Can you work these out from the model? Positions are in its coordinate system, mm. A direction names the side the tool comes from. Round coordinates to 2 decimals unless told otherwise and drop trailing zeros. Order: outer loops, then holes, each group sorted by start corner. A loop starts at its lowest first (then second) coordinate and runs counter-clockwise, first axis right, second up. Notation, with made-up numbers: M 46.25,-24.5 L 82.25,-24.5 A27 cw 82.25,6.5 Z; hole C 43.25,85.5 d8. An arc over 180 degrees is marked long. Answer as a JSON object with one key per item and string values. Group by question number.
```python
from build123d import *

# Parameters (mm, degrees)
SKETCH1_W           = 40
SKETCH1_H           = 40
BOSS_EXTRUDE1_DEPTH = 20
SKETCH2_R           = 2.5
BOSS_EXTRUDE2_DEPTH = 5.522
SKETCH5_R           = 9.990957645
SKETCH5_R_2         = 4.140871972
BOSS_EXTRUDE5_DEPTH = 5.08


with BuildPart() as part:
    # Sketch1 → Boss-Extrude1 (new body)
    with BuildSketch(Plane(origin=(0, 0, 0), x_dir=(1, 0, 0), z_dir=(0, 1, 0))):
        Rectangle(SKETCH1_W, SKETCH1_H)
    extrude(amount=BOSS_EXTRUDE1_DEPTH)

    # Sketch2 → Boss-Extrude2 (add)
    with BuildSketch(Plane(origin=(20, 0, 0), x_dir=(0, 0, -1), z_dir=(1, 0, 0))):
        with Locations(Location((10, 10, 0), (0, 0, 180))):
            Circle(SKETCH2_R)
    boss_extrude2 = extrude(amount=BOSS_EXTRUDE2_DEPTH)

    # Mirror1: Boss-Extrude2 across plane
    add(boss_extrude2.mirror(Plane(origin=(0, 0, 0), x_dir=(0, 0, 1), z_dir=(1, 0, 0))))

    # Sketch5 → Boss-Extrude5 (add)
    with BuildSketch(Plane(origin=(20, 0, 0), x_dir=(0, 0, -1), z_dir=(1, 0, 0))):
        with Locations(Location((10, 10, 0), (0, 0, 180))):
            Circle(SKETCH5_R)
        with Locations((10, 10)):
            Circle(SKETCH5_R_2, mode=Mode.SUBTRACT)
    boss_extrude5 = extrude(amount=BOSS_EXTRUDE5_DEPTH)

    # Mirror2: Boss-Extrude5 across plane
    add(boss_extrude5.mirror(Plane(origin=(0, 0, 0), x_dir=(0, 0, 1), z_dir=(1, 0, 0))))


solid = part.part
```
1) For pin 1 (4 mm diameter, centred on y = 8.5, z = 4, fed in from -X); pin 2 (10 mm diameter, centred on y = 17, z = -14, fed in from +X); pin 3 (3 mm diameter, centred on y = 13, z = 1, fed in from -X), each with a flat end and sliding along its axis, tell me the tip position at first contact or that it passes through.
2) Which directions (+Z, -Z, +X, -X, +Y, -Y) give clear straight access to the entire face, cutting with the end or side of a thin tool? Please do faces 1 (the face through (-25.522, 10, -10)), 2 (the face through (-20, 12, -12)), 3 (the face through (25.08, 14.3, -10.1)).
3) If we section it at A-A on y = 15: Write out the boundary of the cut face in (x, z).
4) We'd pull the mould along Y, two halves only. Please class faces 4 (the face through (0, 0, 0)), 5 (the face through (20, 10, 9)), 6 (the face through (-22.72, 12.44, -10.54)): +Y half, -Y half, draft (parallel to the pull), parting line (faces both ways), or undercut.
5) I need wall thicknesses on line 1 along Y through (x, z) = (22.55, -10); line 2 along X through (y, z) = (1, -2); line 3 along X through (y, z) = (12, -16). Which ranges of each line are inside material? Lowest first, please.
6) If we section it at D-D on z = 1: Write out the boundary of the cut face in (x, y).
Findings:
{
 "1": {"pin 1": "stops at x = -20", "pin 2": "stops at x = 25.08", "pin 3": "stops at x = -25.08"},
 "2": {"face 1": "+Z, -Z, -X, +Y, -Y", "face 2": "-X", "face 3": "+X"},
 "3": {"outline": "M -25.08,-18.65 L -20,-18.65 L -20,-20 L 20,-20 L 20,-18.65 L 25.08,-18.65 L 25.08,-1.35 L 20,-1.35 L 20,20 L -20,20 L -20,-1.35 L -25.08,-1.35 Z"},
 "4": {"face 4": "-Y half", "face 5": "draft", "face 6": "undercut"},
 "5": {"line 1": "y = 0.01 to 5.86, 7.5 to 12.5, 14.14 to 19.99", "line 2": "x = -20 to 20", "line 3": "x = -25.08 to 25.08"},
 "6": {"outline": "M -20,0 L 20,0 L 20,20 L -20,20 Z"}
}
